Work out the finished part from the listing and answer in its coordinate system (mm). Coordinates: 2 decimals unless noted, no trailing zeros. Order: outer loops, then holes, each group sorted by start corner. A loop starts at its lowest first (then second) coordinate and runs counter-clockwise, first axis right, second up. Notation, with made-up numbers: M 29.5,63 L 68.5,63 A16 cw 68.5,69 Z; hole C 6,86 d2. An arc over 180 degrees is marked long. Answer in a Markdown table with one row per item. Add a question column.
Item 1: The mould has two halves that part along X. Classify faces 1 (the face through (3.5, 6.35, 1.4)), 2 (the face through (-3.996, 3.131, 3.136)): released by +X, released by -X, zero draft, split by the parting line, or undercut.
Item 2: Consider line 1 (X direction, y = 1.75, z = 0); line 2 (X direction, y = 1.25, z = -2.75); line 3 (X direction, y = 5.25, z = 4.5). Determine where each line is inside the solid, lowest interval first. Write a range as from..to.
Item 3: The part is cut by section A-A (x = 0). Write down the section's boundary in (y, z).
Item 4: Flat-ended cylindrical pins translate along their axes: pin 1 Ø3 at (x, z) = (6, 3.5) entering from -Y; pin 2 Ø1.5 at (x, y) = (2.5, 1) entering from -Z. Find the tip coordinate at first contact, or state that the pin passes through.
Item 5: The part is cut by section C-C (z = 3). Write down the section's boundary in (x, y).
Item 6: The part is cut by section B-B (y = 2.5). State how many separate pieces and enclosed holes the cut face has, then the cut area to 3 significant figures.
from build123d import *

# Parameters (mm, degrees)
SKETCH1_R           = 3.556
BOSS_EXTRUDE1_DEPTH = 6.35
SKETCH2_R           = 1.651
CUT_EXTRUDE1_DEPTH  = 6.35
FILLET1_R           = 0.0254


with BuildPart() as part:
    # Sketch1 → Boss-Extrude1 (new body)
    with BuildSketch(Plane(origin=(0, 0, 0), x_dir=(1, 0, 0), z_dir=(0, 1, 0))):
        with BuildLine():
            Line((22.365139772, -13.37924688), (15.035220761, -6.343773385))
            Line((15.035220761, -6.343773385), (3.521977792, 3.669378045))
            Line((3.521977792, 3.669378045), (3.517736747, 3.664959506))
            ThreePointArc((3.517736747, 3.664959506), (-3.784384399, -3.388928255), (4.029432062, 3.093554146))
            Line((4.029432062, 3.093554146), (14.964866026, -6.417072576))
            Line((14.964866026, -6.417072576), (22.294785037, -13.45254607))
            Line((22.294785037, -13.45254607), (22.365139772, -13.37924688))
        make_face()
        with Locations(Location((0, 0, 0), (0, 0, 270))):
            Circle(SKETCH1_R, mode=Mode.SUBTRACT)
    extrude(amount=BOSS_EXTRUDE1_DEPTH)

    # Sketch2 → Cut-Extrude1 (cut)
    with BuildSketch(Plane(origin=(3.305454811, 0, -4.914803593), x_dir=(-0.7214487215857361, 0, -0.6924678636025697), z_dir=(0.6924678636025697, 0, -0.7214487215857361))):
        with Locations((-22.608627396, 3.175)):
            Circle(SKETCH2_R)
    extrude(amount=-CUT_EXTRUDE1_DEPTH, mode=Mode.SUBTRACT)

    # Fillet1
    fillet1_edges = [part.edges().sort_by_distance(p)[0] for p in [
        (4.029432062, 3.175, -3.093554146),
    ]]
    fillet(fillet1_edges, radius=FILLET1_R)


solid = part.part
Reply:
| question | item | result |
|---|---|---|
| 1 | face 1 | zero draft |
| 1 | face 2 | undercut |
| 2 | line 1 | x = -5.08..-3.56, 3.56..5.08, 7.59..7.74 |
| 2 | line 2 | x = -4.27..-2.25, 2.25..4.27, 4.42..4.58 |
| 2 | line 3 | x = -2.36..2.36, 12.76..12.92 |
| 3 | outline | M 0,-5.08 L 6.35,-5.08 L 6.35,-3.56 L 0,-3.56 Z; M 0,3.56 L 6.35,3.56 L 6.35,5.08 L 0,5.08 Z |
| 4 | pin 1 | passes through |
| 4 | pin 2 | stops at z = -4.77 |
| 5 | outline | M -4.1,0 L -1.91,0 L -1.91,6.35 L -4.1,6.35 Z; M 1.91,0 L 4.1,0 L 4.1,6.35 L 1.91,6.35 Z; M 11.04,0 L 11.19,0 L 11.19,6.35 L 11.04,6.35 Z |
| 6 | separate pieces | 2 |
| 6 | enclosed holes | 1 |
| 6 | area | 43.6 mm2 |
